Check sheet for the modelled part. Datum: model origin and axes. Units: mm. A direction names the side the tool comes from. Coordinates: 2 decimals unless noted, no trailing zeros. Loops run counter-clockwise (first coordinate to the right, second up) from the corner with the lowest first, then second, coordinate; pieces in that order, holes last. Notation, with made-up numbers: (25, 42.5) - (46, 42.5) arc R28 cw to (46, 78.5) - close; hole circle Ø1 at (88.5, 30.5). An arc over 180 degrees is marked (long way). Use a Markdown table: item, result. Add a question column.
1) Draft check along Y on faces 1 (the flat face through (-59, 2, 59)), 2 (the flat face through (-10, 50.2, 39)), 3 (the flat face through (-35, 35, 14)), 4 (the flat face through (-65, 62, 64)). Enter one of: pulls with the +Y half, pulls with the -Y half, needs draft (parallel to the pull), parting line crosses it, or undercut.
2) Thickness scan on line 1 (X direction, y = 60.1, z = 26); line 2 (Y direction, x = -16, z = 43.5); line 3 (X direction, y = 58, z = 58.5). Record the ranges inside material, lowest first.
3) Sectioned sample at A-A, the plane z = 49. Enter the section's corners in (x, y), then the cut area to 3 significant figures.
4) Go/stop test with flat-tipped pins: P1, Ø1.5, axis at x = -7.5, z = 59.5, coming from the -Y side; P2, Ø1, axis at x = -22, z = 49, coming from the -Y side; P3, Ø1.5, axis at x = -60.5, z = 60, coming from the +Y side; P4, Ø10, axis at x = -35.5, y = 46.5, coming from the +Z side. Record where each tip stops, or that it passes through.
5) Sectioned sample at C-C, the plane y = 9.9. Enter the section's corners in (x, z).
6) Sectioned sample at B-B, the plane x = -60.1. Enter the section's corners in (y, z), then the cut area to 3 significant figures.
7) Tool access check on faces 5 (the flat face through (-10, 68, 59)), 6 (the flat face through (-60, 19.8, 39)), 7 (the flat face through (-68.2, 64.5, 61)), 8 (the flat face through (-68, 11, 60)), 9 (the flat face through (-10, 2, 59)). Record the directions out of +Z, -Z, +X, -X, +Y, -Y that give a thin tool (end or side, any length) a straight path to the whole face; none if there is none.
8) Sectioned sample at D-D, the plane z = 8.5. Enter the section's corners in (x, y), then the cut area to 3 significant figures.
from build123d import *

# Parameters (mm, degrees)
ESQUISSE1_W                  = 70
ESQUISSE1_H                  = 70
BOSS_EXTRU_1_DEPTH           = 64
ESQUISSE2_W                  = 30.4
ESQUISSE2_H                  = 19.8
ESQUISSE2_H_2                = 30.4
ESQUISSE2_W_2                = 19.8
ENL_V_MAT_EXTRU_1_DEPTH      = 50
ESQUISSE5_W                  = 3
ESQUISSE5_H                  = 2
ENL_V_MAT_EXTRU_3_DEPTH      = 71
ESQUISSE6_W                  = 2
ESQUISSE6_H                  = 3
ENL_V_MAT_EXTRU_4_DEPTH      = 71
ESQUISSE7_R                  = 5
ENL_V_MAT_EXTRU_5_DEPTH      = 65
R_P_TITION_CIRCULAIRE2_COUNT = 4


with BuildPart() as part:
    # Esquisse1 → Boss.-Extru.1 (new body)
    with BuildSketch(Plane.XY):
        with Locations((-35, 35)):
            Rectangle(ESQUISSE1_W, ESQUISSE1_H)
    extrude(amount=BOSS_EXTRU_1_DEPTH)

    # Esquisse2 → Enlèv. mat.-Extru.1 (cut)
    with BuildSketch(Plane.XY.offset(64)):
        with Locations((-35, 60.1)):
            Rectangle(ESQUISSE2_W, ESQUISSE2_H)
        with Locations((-35, 35)):
            Rectangle(ESQUISSE2_W, ESQUISSE2_H_2)
        with Locations((-9.9, 35)):
            Rectangle(ESQUISSE2_W_2, ESQUISSE2_H_2)
        with Locations((-60.1, 35)):
            Rectangle(ESQUISSE2_W_2, ESQUISSE2_H_2)
        with Locations((-35, 9.9)):
            Rectangle(ESQUISSE2_W, ESQUISSE2_H)
    extrude(amount=-ENL_V_MAT_EXTRU_1_DEPTH, mode=Mode.SUBTRACT)

    # Esquisse5 → Enlèv. mat.-Extru.3 (cut, through all)
    with BuildSketch(Plane.ZY.offset(70)):
        with Locations((59.5, 69)):
            Rectangle(ESQUISSE5_W, ESQUISSE5_H)
        with Locations((59.5, 1)):
            Rectangle(ESQUISSE5_W, ESQUISSE5_H)
    extrude(amount=-ENL_V_MAT_EXTRU_3_DEPTH, mode=Mode.SUBTRACT)

    # Esquisse6 → Enlèv. mat.-Extru.4 (cut, through all)
    with BuildSketch(Plane(origin=(0, 70, 0), x_dir=(1, 0, 0), z_dir=(0, 1, 0))):
        with Locations((-69, -59.5)):
            Rectangle(ESQUISSE6_W, ESQUISSE6_H)
    extrude(amount=-ENL_V_MAT_EXTRU_4_DEPTH, mode=Mode.SUBTRACT)

    # Esquisse7 → Enlèv. mat.-Extru.5 (cut, through all)
    with BuildSketch(Plane.XY.offset(64)):
        with Locations((-9.9, 9.9)):
            Circle(ESQUISSE7_R)
    enl_v_mat_extru_5 = extrude(amount=-ENL_V_MAT_EXTRU_5_DEPTH, mode=Mode.SUBTRACT)

    # Répétition circulaire2: Enlèv. mat.-Extru.5 ×4 about axis
    r_p_tition_circulaire2_axis = Axis((-35, 35, 0), (0, 0, 1))
    for i in range(1, R_P_TITION_CIRCULAIRE2_COUNT):
        add(enl_v_mat_extru_5.rotate(r_p_tition_circulaire2_axis, i * 360 / R_P_TITION_CIRCULAIRE2_COUNT), mode=Mode.SUBTRACT)


solid = part.part
Solved:
| question | item | result |
|---|---|---|
| 1 | face 1 | pulls with the -Y half |
| 1 | face 2 | undercut |
| 1 | face 3 | undercut |
| 1 | face 4 | needs draft |
| 2 | line 1 | x = -70 to -65.1, -55.1 to -50.2, -19.8 to -14.9, -4.9 to 0 |
| 2 | line 2 | y = 0 to 19.8, 50.2 to 70 |
| 2 | line 3 | x = -68 to -64.64, -55.56 to -50.2, -19.8 to -14.44, -5.36 to 0 |
| 3 | outline | (-70, 0) - (-50.2, 0) - (-50.2, 19.8) - (-70, 19.8) - close; (-70, 50.2) - (-50.2, 50.2) - (-50.2, 70) - (-70, 70) - close; (-19.8, 0) - (0, 0) - (0, 19.8) - (-19.8, 19.8) - close; (-19.8, 50.2) - (0, 50.2) - (0, 70) - (-19.8, 70) - close; hole circle Ø10 at (-60.1, 9.9); hole circle Ø10 at (-60.1, 60.1); hole circle Ø10 at (-9.9, 9.9); hole circle Ø10 at (-9.9, 60.1) |
| 3 | area | 1,250 mm2 |
| 4 | P1 | stops at y = 2 |
| 4 | P2 | passes through |
| 4 | P3 | stops at y = 68 |
| 4 | P4 | stops at z = 14 |
| 5 | outline | (-70, 0) - (-65.1, 0) - (-65.1, 64) - (-70, 64) - (-70, 61) - (-68, 61) - (-68, 58) - (-70, 58) - close; (-55.1, 0) - (-14.9, 0) - (-14.9, 64) - (-19.8, 64) - (-19.8, 14) - (-50.2, 14) - (-50.2, 64) - (-55.1, 64) - close; (-4.9, 0) - (0, 0) - (0, 64) - (-4.9, 64) - close |
| 6 | outline | (0, 0) - (4.9, 0) - (4.9, 64) - (0, 64) - (0, 61) - (2, 61) - (2, 58) - (0, 58) - close; (14.9, 0) - (55.1, 0) - (55.1, 64) - (50.2, 64) - (50.2, 14) - (19.8, 14) - (19.8, 64) - (14.9, 64) - close; (65.1, 0) - (70, 0) - (70, 58) - (68, 58) - (68, 61) - (70, 61) - (70, 64) - (65.1, 64) - close |
| 6 | area | 1,670 mm2 |
| 7 | face 5 | +X, -X, +Y |
| 7 | face 6 | +Z, +X, -X |
| 7 | face 7 | -X, +Y |
| 7 | face 8 | -X, +Y, -Y |
| 7 | face 9 | +X, -X, -Y |
| 8 | outline | (-70, 0) - (0, 0) - (0, 70) - (-70, 70) - close; hole circle Ø10 at (-60.1, 9.9); hole circle Ø10 at (-60.1, 60.1); hole circle Ø10 at (-9.9, 9.9); hole circle Ø10 at (-9.9, 60.1) |
| 8 | area | 4,590 mm2 |
